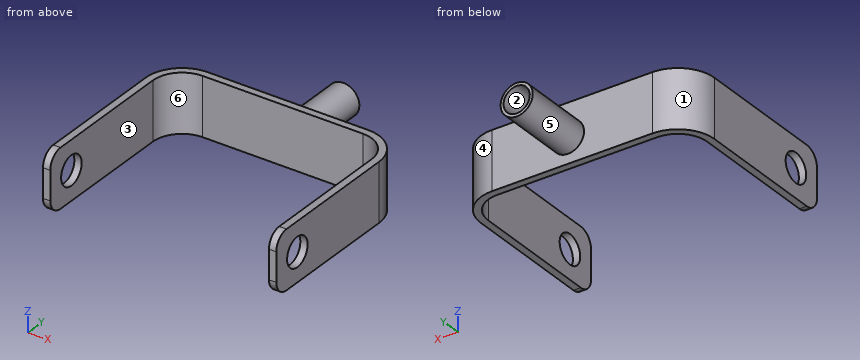
from build123d import *

# Parameters (mm, degrees)
BASE_FLANGE1_DEPTH  = 40
FILLET1_R           = 10
SKETCH3_R           = 10
CUT_EXTRUDE1_DEPTH  = 207.942020866
SKETCH4_R           = 11
SKETCH4_R_2         = 9
BOSS_EXTRUDE1_DEPTH = 50


# Sheet-metal steps are written as plain solids
with BuildPart() as part:
    # Sketch1 → Base-Flange1 (new body)
    with BuildSketch(Plane.XY):
        with BuildLine():
            Line((0, 0), (0, 100))
            ThreePointArc((0, 100), (5.857864376, 114.142135624), (20, 120))
            Line((20, 120), (130, 120))
            ThreePointArc((130, 120), (144.142135624, 114.142135624), (150, 100))
            Line((150, 100), (150, 0))
            Line((150, 0), (155, 0))
            Line((155, 0), (155, 100))
            ThreePointArc((155, 100), (147.67766953, 117.67766953), (130, 125))
            Line((130, 125), (20, 125))
            ThreePointArc((20, 125), (2.32233047, 117.67766953), (-5, 100))
            Line((-5, 100), (-5, 0))
            Line((-5, 0), (0, 0))
        make_face()
    extrude(amount=BASE_FLANGE1_DEPTH)

    # Fillet1
    fillet1_edges = [part.edges().sort_by_distance(p)[0] for p in [
        (152.5, 0, 0),
        (-2.5, 0, 0),
        (152.5, 0, 40),
        (-2.5, 0, 40),
    ]]
    fillet(fillet1_edges, radius=FILLET1_R)

    # Sketch3 → Cut-Extrude1 (cut, through all)
    with BuildSketch(Plane(origin=(155, 0, 0), x_dir=(0, 0, -1), z_dir=(1, 0, 0))):
        with Locations((-19.918118103, 20.545243048)):
            Circle(SKETCH3_R)
    extrude(amount=-CUT_EXTRUDE1_DEPTH, mode=Mode.SUBTRACT)

    # Sketch4 → Boss-Extrude1 (add)
    with BuildSketch(Plane(origin=(0, 125, 0), x_dir=(1, 0, 0), z_dir=(0, 1, 0))):
        with Locations(Location((77.803452919, -17.50804185, 0), (0, 0, 90))):
            Circle(SKETCH4_R)
        with Locations(Location((77.803452919, -17.50804185, 0), (0, 0, 270))):
            Circle(SKETCH4_R_2, mode=Mode.SUBTRACT)
    extrude(amount=BOSS_EXTRUDE1_DEPTH)


solid = part.part
Here's how the part is built. I have some questions about the finished solid (model axes, mm). Face numbers are marked on the shaded views. A direction names the side the tool comes from. Coordinates: 2 decimals unless noted, no trailing zeros. Write each loop counter-clockwise with the first axis right and the second up, starting at its lowest first coordinate (ties: lowest second). Pieces come first, ordered by that corner, then holes.
1) If we section it at A-A (y = 41): List the corners of the cut face in (x, z) for me, plus the area to 3 significant figures.
Filled in:
outline: (-5, 0) - (0, 0) - (0, 40) - (-5, 40) - close; (150, 0) - (155, 0) - (155, 40) - (150, 40) - close
area: 400 mm2
2) If we section it at B-B (y = 17): List the corners of the cut face in (x, z) for me.
Filled in:
outline: (-5, 0) - (0, 0) - (0, 10.57) - (-5, 10.57) - close; (-5, 29.27) - (0, 29.27) - (0, 40) - (-5, 40) - close; (150, 0) - (155, 0) - (155, 10.57) - (150, 10.57) - close; (150, 29.27) - (155, 29.27) - (155, 40) - (150, 40) - close
3) If I drill on line 1 (X direction, y = 87.5, z = 3); line 2 (Y direction, x = 37.5, z = 38); line 3 (X direction, y = 152, z = 22), over which ranges is the centre line in solid material (lowest first)?
Filled in:
line 1: x = -5 to 0, 150 to 155
line 2: y = 120 to 125
line 3: x = 67.76 to 70, 85.6 to 87.84
4) Thinking about a two-plate mould opening in X: for the marked faces 4, 5 and 6, which applies, +X half, -X half, draft (parallel to the pull), parting line (faces both ways), or undercut?
Filled in:
face 4: +X half
face 5: parting line
face 6: undercut
5) I'm going to push flat-ended pins straight in: pin 1 (2 mm diameter, centred on x = 131, z = 6, fed in from +Y); pin 2 (4 mm diameter, centred on y = 129.5, z = 17, fed in from +X); pin 3 (20 mm diameter, centred on x = 77.5, z = 28, fed in from -Y). Where does each tip first touch, or does it pass through?
Filled in:
pin 1: stops at y = 125
pin 2: stops at x = 88.8
pin 3: stops at y = 120
6) If we section it at C-C (z = 4): List the corners of the cut face in (x, y) for me.
Filled in:
outline: (-5, 2) - (0, 2) - (0, 100) arc R20 cw to (20, 120) - (130, 120) arc R20 cw to (150, 100) - (150, 2) - (155, 2) - (155, 100) arc R25 ccw to (130, 125) - (20, 125) arc R25 ccw to (-5, 100) - close
7) If we section it at D-D (x = 56.5): List the corners of the cut face in (y, z) for me.
Filled in:
outline: (120, 0) - (125, 0) - (125, 40) - (120, 40) - close
8) Which directions (+Z, -Z, +X, -X, +Y, -Y) give clear straight access to the entire face, cutting with the end or side of a thin tool? Please do the marked faces 1, 2 and 3.
Filled in:
face 1: +Z, -Z, -X, +Y
face 2: +Y
face 3: +Z, -Z, -Y
